Here's how the part is built. I have some questions about the finished solid (model axes, mm). A direction names the side the tool comes from. Give positions to 0.01 mm unless a question says otherwise; leave off trailing zeros. Order: outer loops, then holes, each group sorted by start corner. A loop starts at its lowest first (then second) coordinate and runs counter-clockwise, first axis right, second up. Notation, with made-up numbers: M -35.75,-31.75 L -23.75,-31.75 A20 ccw -23.75,-3.75 Z; hole C 7.5,-35.5 d1. An arc over 180 degrees is marked long. Use one line per item in the form item = value.
Autodesk Inventor part; units mm, degrees
ref_plane "YZ Plane" through (0, 0, 0) normal (1, 0, 0) x (0, 1, 0)
ref_plane "XZ Plane" through (0, 0, 0) normal (0, 1, 0) x (-1, 0, 0)
ref_plane "XY Plane" through (0, 0, 0) normal (0, 0, 1) x (1, 0, 0)
sketch "Skizze1" plane through (0, 0, 0) normal (0, 1, 0) x (-1, 0, 0)
  line L0 (0, 3) -> (9.5, 3)
  line L1 (9.5, 3) -> (9.5, -3)
  line L2 (9.5, -3) -> (0, -3)
  line L3 (0, -3) -> (0, 3)
  point P0 (0, 0)
  point P1 (0, 0)
  dimension "d0" = 6
  dimension "d1" = 9.5
extrude "Extrusion1" add sketch "Skizze1" along normal blind 8
fillet "Rundung1" radius 3 2 edges at (-9.5, 4, -3) (-9.5, 4, 3)
sketch "Skizze5" plane through (0, 8, 0) normal (0, 1, 0) x (1, 0, 0)
  arc A0 (-6.5, 3) -> (-6.5, -3) centre (-6.5, 0) ccw
  point P0 (0, 0)
hole "Bohrung2" at (-6.5, 8, 0) direction (0, -1, 0) diameter 2 depth 8
sketch "Skizze3" plane through (0, 0, -3) normal (0, 0, -1) x (-1, 0, 0)
  line L0 (3, 6) -> (11.5, 6)
  line L1 (11.5, 6) -> (11.5, 2)
  line L2 (11.5, 2) -> (3, 2)
  line L3 (3, 2) -> (3, 6)
  line L4 (9.5, 0) -> (9.5, 8)
  line L5 (0, 0) -> (0, 8)
  point P0 (3, 4)
  point P1 (0, 4)
  point P2 (7.25, 2)
  point P3 (11.5, 4)
  dimension "d12" = 6.5
  dimension "d13" = 4
  dimension "d14" = 2
extrude "Extrusion2" cut sketch "Skizze3" against normal up to surface (6 mm away)
sketch "Skizze4" plane through (0, 0, 3) normal (1, 0, 0) x (0, 0, -1)
  circle A0 centre (3, 4) radius 1.5
  line L0 (6, 0) -> (6, 8)
  line L1 (0, 0) -> (6, 0)
  point P0 (3, 0)
  point P1 (6, 4)
  point P2 (3, 0)
  dimension "d17" = 3
extrude "Extrusion3" add sketch "Skizze4" along normal blind 5
thread "Gewinde1"
properties part number "top_pleuel"
Q1. I want a section at B-B on x = -4. Write out the boundary of the cut face in (y, z), then the cut area to 3 significant figures.
Found:
outline = M 0,-3 L 2,-3 L 2,3 L 0,3 Z; M 6,-3 L 8,-3 L 8,3 L 6,3 Z
area = 24.0 mm²
Q2. On a 3-axis mill with a long thin cutter (end or side, diameter ignored), from which of +Z, -Z, +X, -X, +Y, -Y can I reach the whole of each face in a straight line? I mean faces 5 (the face through (-8.64, 1.01, 2.1)), 6 (the face through (-5, 6, 0)). Say none if no direction works.
Found:
face_5 = +Z, -X, +Y, -Y
face_6 = +Z, -Z, -X
Q3. I want a section at C-C on z = 0.5. Write out the boundary of the cut face in (x, y), then the cut area to 3 significant figures.
Found:
outline = M -9.46,0 L -7.37,0 L -7.37,2 L -9.46,2 Z; M -9.46,6 L -7.37,6 L -7.37,8 L -9.46,8 Z; M -5.63,0 L 0,0 L 0,2.59 L 5,2.59 L 5,5.41 L 0,5.41 L 0,8 L -5.63,8 L -5.63,6 L -3,6 L -3,2 L -5.63,2 Z
area = 57.0 mm²
Q4. I want a section at D-D on y = 4. Write out the boundary of the cut face in (x, z), then the cut area to 3 significant figures.
Found:
outline = M -3,-3 L 0,-3 L 0,-1.5 L 5,-1.5 L 5,1.5 L 0,1.5 L 0,3 L -3,3 Z
area = 33.0 mm²
Q5. I'm going to push flat-ended pins straight in: pin 1 Ø2 at (y, z) = (3.5, 0) entering from -X; pin 2 Ø4 at (x, y) = (2.5, 2.5) entering from -Z; pin 3 Ø1.2 at (x, z) = (-6.5, 0) entering from +Y. Where does each tip first touch, or does it pass through?
Found:
pin_1 = -3
pin_2 = -1.5
pin_3 = through
Q6. I need wall thicknesses on L1, parallel to X at y = 6.6, z = 0; L2, parallel to Y at x = -7.75, z = -0.6; L3, parallel to Z at x = -6.5, y = 7.1. Which ranges of each line are inside material? Lowest first, please.
Found:
L1 = -9.5 to -7.5, -5.5 to 0
L2 = 0 to 2, 6 to 8
L3 = -3 to -1, 1 to 3
Q7. Thinking about a two-plate mould opening in Z: for faces 1 (the face through (-2, 4, 3)), 2 (the face through (2.465, 2.513, 0.195)), 3 (the face through (-7.49, 6.99, -0.13)), 4 (the face through (-8.6, 7.01, -2.14)), which applies, +Z half, -Z half, draft (parallel to the pull), parting line (faces both ways), or undercut?
Found:
face_1 = +Z half
face_2 = parting line
face_3 = undercut
face_4 = -Z half
